```python
from build123d import *

# Parameters (mm, degrees)
SKETCH1_R           = 9.25
BOSS_EXTRUDE1_DEPTH = 42
SKETCH2_R           = 10.31875
CUT_EXTRUDE1_DEPTH  = 11.1125
SKETCH3_R           = 10.3175
CUT_EXTRUDE2_DEPTH  = 11.1125
CUT_EXTRUDE3_DEPTH  = 19.775
SKETCH5_R           = 3
CUT_EXTRUDE4_DEPTH  = 8
SKETCH6_W           = 19
SKETCH6_H           = 20
CUT_EXTRUDE5_DEPTH  = 6
FILLET1_R           = 2.38


with BuildPart() as part:
    # Sketch1 → Boss-Extrude1 (new body)
    with BuildSketch(Plane(origin=(0, 0, 0), x_dir=(1, 0, 0), z_dir=(0, 1, 0))):
        with BuildLine():
            Line((-13.31875, 0), (-13.31875, 13.31875))
            Line((-13.31875, 13.31875), (-13.31875, 17.81875))
            Line((-13.31875, 17.81875), (-13.31875, 18.81875))
            Line((-13.31875, 18.81875), (13.31875, 18.81875))
            Line((13.31875, 18.81875), (13.31875, 17.81875))
            Line((13.31875, 17.81875), (13.31875, 13.31875))
            Line((13.31875, 13.31875), (13.31875, 0))
            ThreePointArc((13.31875, 0), (0, -13.31875), (-13.31875, 0))
        make_face()
        with Locations(Location((0, 0, 0), (0, 0, 90))):
            Circle(SKETCH1_R, mode=Mode.SUBTRACT)
    extrude(amount=BOSS_EXTRUDE1_DEPTH)

    # Sketch2 → Cut-Extrude1 (cut)
    with BuildSketch(Plane(origin=(0, 42, 0), x_dir=(1, 0, 0), z_dir=(0, 1, 0))):
        with Locations(Location((0, 0, 0), (0, 0, 270))):
            Circle(SKETCH2_R)
    extrude(amount=-CUT_EXTRUDE1_DEPTH, mode=Mode.SUBTRACT)

    # Sketch3 → Cut-Extrude2 (cut)
    with BuildSketch(Plane.XZ):
        with Locations(Location((0, 0, 0), (0, 0, 270))):
            Circle(SKETCH3_R)
    extrude(amount=-CUT_EXTRUDE2_DEPTH, mode=Mode.SUBTRACT)

    # Sketch4 → Cut-Extrude3 (cut)
    with BuildSketch(Plane(origin=(0, 30.8875, 0), x_dir=(1, 0, 0), z_dir=(0, 1, 0))):
        Polygon((2.702073717, -6.203740676), (-2.702073717, -6.203740676), (-2.702073717, -16.08189807), (-18.957765954, -16.08189807), (-18.957765954, 3.606897718), (22.504521647, 3.606897718), (22.504521647, -16.08189807), (2.702073717, -16.08189807), align=None)
    extrude(amount=-CUT_EXTRUDE3_DEPTH, mode=Mode.SUBTRACT)

    # Sketch5 → Cut-Extrude4 (cut)
    with BuildSketch(Plane(origin=(0, 0, -18.81875), x_dir=(-1, 0, 0), z_dir=(0, 0, -1))):
        with Locations((-7.81875, 5.5)):
            Circle(SKETCH5_R)
        with Locations((7.81875, 5.5)):
            Circle(SKETCH5_R)
        with Locations((7.81875, 36.5)):
            Circle(SKETCH5_R)
        with Locations((-7.81875, 36.5)):
            Circle(SKETCH5_R)
    extrude(amount=-CUT_EXTRUDE4_DEPTH, mode=Mode.SUBTRACT)

    # Sketch6 → Cut-Extrude5 (cut)
    with BuildSketch(Plane(origin=(0, 0, -18.81875), x_dir=(-1, 0, 0), z_dir=(0, 0, -1))):
        with Locations((0, 21)):
            Rectangle(SKETCH6_W, SKETCH6_H)
    extrude(amount=-CUT_EXTRUDE5_DEPTH, mode=Mode.SUBTRACT)

    # Fillet1
    fillet1_edges = [part.edges().sort_by_distance(p)[0] for p in [
        (-9.5, 31, -15.81875),
        (-9.5, 11, -15.81875),
        (9.5, 11, -15.81875),
        (9.5, 31, -15.81875),
    ]]
    fillet(fillet1_edges, radius=FILLET1_R)


solid = part.part
```
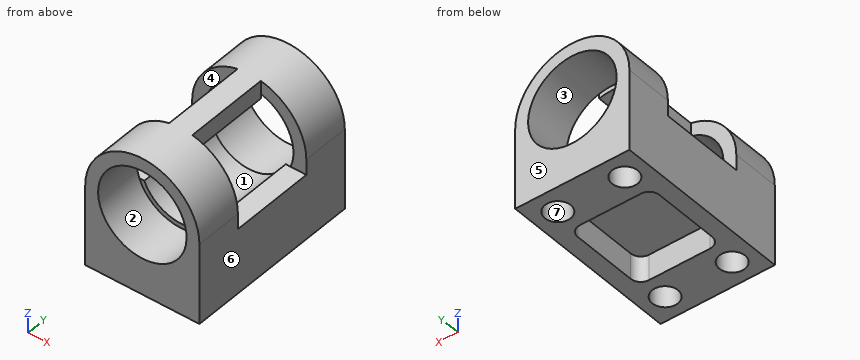
Input: part model. Units: mm. Frame: model coordinates. Face numbers are marked on the shaded views. A direction names the side the tool comes from. Round coordinates to 2 decimals unless told otherwise and drop trailing zeros. Loops run counter-clockwise (first coordinate to the right, second up) from the corner with the lowest first, then second, coordinate; pieces in that order, holes last. Notation, with made-up numbers: (81, -39) -> (99, -39) arc R21 cw to (99, -23) -> close; hole circle Ø11 at (30.25, -36.5). An arc over 180 degrees is marked (long way). Use one line per item in the form item = value. Start each with the question number.
Item 1: Section query D-D on y = 14.5. Return the cut outline in (x, z).
Item 2: Section query A-A on x = 0. Return the cut outline in (y, z).
Item 3: Mould query, pull axis X, two halves, no side actions, for the marked faces 5, 6 and 7. Classes: pulls with the +X half, pulls with the -X half, needs draft (parallel to the pull), parting line crosses it, or undercut.
Item 4: Contact query for flat-ended pins moving along their axis: pin 1 Ø2 at (x, z) = (-9, -10.5) entering from -Y; pin 2 Ø8 at (x, y) = (-7.82, 36.5) entering from +Z; pin 3 Ø2 at (x, y) = (2, 35.5) entering from +Z; pin 4 Ø1.3 at (y, z) = (22, 11.5) entering from +X. Output: stop coordinate, or through.
Item 5: Set-up query: the marked faces 1, 2, 3 and 4. Return all of +Z, -Z, +X, -X, +Y, -Y with unobstructed straight access to the full face (end or side cutting, diameter ignored); none if empty.
Item 6: Section query C-C on z = -14. Return the cut outline in (x, y).
Item 7: Section query B-B on y = 5.5. Return the cut outline in (x, z) (1 decimal).
Item 8: Material intervals for L1, parallel to Y at x = -11.25, z = 5.5; L2, parallel to Y at x = -9.75, z = -12.5; L3, parallel to X at y = 40.5, z = 7.5, sorted ascending. Write a range as from..to.
Ans:
q1.outline = (-13.32, -18.82) -> (-9.5, -18.82) -> (-9.5, -12.82) -> (9.5, -12.82) -> (9.5, -18.82) -> (13.32, -18.82) -> (13.32, -3.61) -> (8.52, -3.61) arc R9.25 cw to (-8.52, -3.61) -> (-13.32, -3.61) -> close; (-2.7, 8.85) arc R9.25 cw to (2.7, 8.85) -> (2.7, 13.04) arc R13.32 ccw to (-2.7, 13.04) -> close
q2.outline = (0, -18.82) -> (11, -18.82) -> (11, -12.82) -> (31, -12.82) -> (31, -18.82) -> (42, -18.82) -> (42, -10.32) -> (30.89, -10.32) -> (30.89, -9.25) -> (11.11, -9.25) -> (11.11, -10.32) -> (0, -10.32) -> close; (0, 10.32) -> (11.11, 10.32) -> (11.11, 9.25) -> (30.89, 9.25) -> (30.89, 10.32) -> (42, 10.32) -> (42, 13.32) -> (0, 13.32) -> close
q3.face_5 = needs draft
q3.face_6 = pulls with the +X half
q3.face_7 = undercut
q4.pin_1 = 0
q4.pin_2 = 12.76
q4.pin_3 = 13.28
q4.pin_4 = 2.7
q5.face_1 = +Y, -Y
q5.face_2 = -Y
q5.face_3 = +Y
q5.face_4 = +Z, -X
q6.outline = (-13.32, 0) -> (13.32, 0) -> (13.32, 42) -> (-13.32, 42) -> close; hole circle Ø6 at (-7.82, 5.5); hole circle Ø6 at (-7.82, 36.5); hole (-9.5, 13.38) arc R2.38 ccw to (-7.12, 11) -> (7.12, 11) arc R2.38 ccw to (9.5, 13.38) -> (9.5, 28.62) arc R2.38 ccw to (7.12, 31) -> (-7.12, 31) arc R2.38 ccw to (-9.5, 28.62) -> close; hole circle Ø6 at (7.82, 5.5); hole circle Ø6 at (7.82, 36.5)
q7.outline = (-13.3, -18.8) -> (-10.8, -18.8) -> (-10.8, -10.8) -> (-4.8, -10.8) -> (-4.8, -18.8) -> (4.8, -18.8) -> (4.8, -10.8) -> (10.8, -10.8) -> (10.8, -18.8) -> (13.3, -18.8) -> (13.3, 0) arc R13.3 ccw to (-13.3, 0) -> close; hole circle Ø20.6 at (0, 0)
q8.L1 = 0..11.11, 30.89..42
q8.L2 = 0..3.2, 7.8..34.2, 38.8..42
q8.L3 = -11.01..-7.09, 7.09..11.01
